from build123d import *
from OCP.BRepFilletAPI import BRepFilletAPI_MakeChamfer

# Parameters (mm, degrees)
SKETCH1_W                = 50
SKETCH1_H                = 21
BOSS_EXTRUDE1_DEPTH      = 2
SKETCH2_W                = 50
SKETCH2_H                = 42
SKETCH2_R                = 2
SKETCH2_R_2              = 12.5
BOSS_EXTRUDE2_DEPTH      = 4
BOSS_EXTRUDE3_START      = -50
BOSS_EXTRUDE3_DEPTH      = 50
CUT_EXTRUDE1_START       = -17
SKETCH4_W                = 46
SKETCH4_H                = 40
CUT_EXTRUDE1_DEPTH       = 17
BOSS_EXTRUDE4_DEPTH      = 8
BOSS_EXTRUDE4_DEPTH_BACK = 8
SKETCH6_R                = 12.5
CUT_EXTRUDE2_DEPTH       = 68.475921631
CHAMFER1_SIZE            = 1
CHAMFER1_SIZE2           = 1.795054936
CHAMFER2_SIZE            = 2


with BuildPart() as part:
    # Sketch1 → Boss-Extrude1 (new body)
    with BuildSketch(Plane(origin=(0, 0, 0), x_dir=(1, 0, 0), z_dir=(0, 1, 0))):
        with Locations((25, 10.5)):
            Rectangle(SKETCH1_W, SKETCH1_H)
        with BuildLine():
            Line((7.25, 11), (7.25, 10))
            ThreePointArc((7.25, 10), (5, 7.75), (2.75, 10))
            Line((2.75, 10), (2.75, 11))
            ThreePointArc((2.75, 11), (5, 13.25), (7.25, 11))
        make_face(mode=Mode.SUBTRACT)
        with BuildLine():
            Line((42.75, 11), (42.75, 10))
            ThreePointArc((42.75, 10), (45, 7.75), (47.25, 10))
            Line((47.25, 10), (47.25, 11))
            ThreePointArc((47.25, 11), (45, 13.25), (42.75, 11))
        make_face(mode=Mode.SUBTRACT)
        with BuildLine():
            Line((27.25, 16), (27.25, 15))
            ThreePointArc((27.25, 15), (25, 12.75), (22.75, 15))
            Line((22.75, 15), (22.75, 16))
            ThreePointArc((22.75, 16), (25, 18.25), (27.25, 16))
        make_face(mode=Mode.SUBTRACT)
    extrude(amount=BOSS_EXTRUDE1_DEPTH)

    # Sketch2 → Boss-Extrude2 (add)
    with BuildSketch(Plane.XY):
        with Locations((25, 21)):
            Rectangle(SKETCH2_W, SKETCH2_H)
        with Locations((9.5, 36.5)):
            Circle(SKETCH2_R, mode=Mode.SUBTRACT)
        with Locations((9.5, 5.5)):
            Circle(SKETCH2_R, mode=Mode.SUBTRACT)
        with Locations((40.5, 5.5)):
            Circle(SKETCH2_R, mode=Mode.SUBTRACT)
        with Locations((40.5, 36.5)):
            Circle(SKETCH2_R, mode=Mode.SUBTRACT)
        with Locations((25, 21)):
            Circle(SKETCH2_R_2, mode=Mode.SUBTRACT)
    extrude(amount=-BOSS_EXTRUDE2_DEPTH)

    # Sketch3 → Boss-Extrude3 (add)
    with BuildSketch(Plane(origin=(50, 0, 0), x_dir=(0, 0, -1), z_dir=(1, 0, 0)).offset(BOSS_EXTRUDE3_START)):
        with BuildLine():
            Line((21, 2), (4, 42))
            Line((4, 42), (4, 2))
            Line((4, 2), (6.5, 2))
            Line((6.5, 2), (6.5, 4))
            ThreePointArc((6.5, 4), (6.939339828, 5.060660172), (8, 5.5))
            Line((8, 5.5), (13, 5.5))
            ThreePointArc((13, 5.5), (14.060660172, 5.060660172), (14.5, 4))
            Line((14.5, 4), (14.5, 2))
            Line((14.5, 2), (21, 2))
        make_face()
    extrude(amount=BOSS_EXTRUDE3_DEPTH)

    # Sketch4 → Cut-Extrude1 (cut)
    with BuildSketch(Plane(origin=(0, 0, -21), x_dir=(-1, 0, 0), z_dir=(0, 0, -1)).offset(CUT_EXTRUDE1_START)):
        with Locations((-25, 22)):
            Rectangle(SKETCH4_W, SKETCH4_H)
    extrude(amount=CUT_EXTRUDE1_DEPTH, mode=Mode.SUBTRACT)

    # Sketch5 → Boss-Extrude4 (add, two sides: drawn at the far end of the back side and taken through both)
    with BuildSketch(Plane.ZY.offset(-25).offset(-BOSS_EXTRUDE4_DEPTH_BACK)):
        Polygon((-4, 2), (-8, 2), (-4, 12), align=None)
    extrude(amount=BOSS_EXTRUDE4_DEPTH + BOSS_EXTRUDE4_DEPTH_BACK)

    # Sketch6 → Cut-Extrude2 (cut, through all)
    with BuildSketch(Plane.XY.offset(-4)):
        with Locations((25, 21)):
            Circle(SKETCH6_R)
    extrude(amount=-CUT_EXTRUDE2_DEPTH, mode=Mode.SUBTRACT)

    # Chamfer1: one chamfer whose edges measure the first distance from different faces: ONE call of the kernel's chamfer builder (chamfer() names one face for all edges)
    chamfer1_edges_1 = [part.edges().sort_by_distance(p)[0] for p in [
        (2, 2, -17.75),
        (48, 2, -17.75),
        (48, 2, -5.25),
        (40.5, 2, -4),
        (2, 2, -5.25),
        (9.5, 2, -4),
        (33, 2, -6),
        (17, 2, -6),
    ]]
    chamfer1_edges_2 = [part.edges().sort_by_distance(p)[0] for p in [
        (25, 2, -8),
    ]]
    chamfer1_side_2 = [part.faces().sort_by_distance(p)[0] for p in [
        (1, 2, -13.971890163),
    ]]
    chamfer1 = BRepFilletAPI_MakeChamfer(part.part.solid().wrapped)
    for e in chamfer1_edges_1:
        chamfer1.Add(CHAMFER1_SIZE, e.wrapped)
    for e in chamfer1_edges_2:
        chamfer1.Add(CHAMFER1_SIZE, CHAMFER1_SIZE2, e.wrapped, chamfer1_side_2[0].wrapped)  # the first distance lies on this face
    add(Compound.cast(chamfer1.Shape()), mode=Mode.REPLACE)

    # Chamfer2
    chamfer2_edges = [part.edges().sort_by_distance(p)[0] for p in [
        (48, 22.5, -4),
        (2, 22.5, -4),
    ]]
    chamfer(chamfer2_edges, length=CHAMFER2_SIZE - 0.0001)  # a hair under: the kernel refuses the full size


solid = part.part
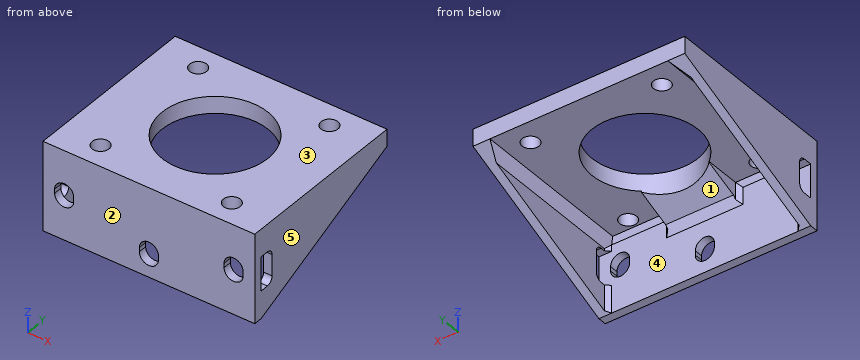
Input: part model. Units: mm. Frame: model coordinates. Face numbers are marked on the shaded views. A direction names the side the tool comes from. Give positions to 0.01 mm unless a question says otherwise; leave off trailing zeros. Order: outer loops, then holes, each group sorted by start corner. A loop starts at its lowest first (then second) coordinate and runs counter-clockwise, first axis right, second up. Notation, with made-up numbers: M 13.25,8 L 62.25,8 A12 cw 62.25,19 Z; hole C 66,4.5 d1. An arc over 180 degrees is marked long. Answer as a JSON object with one key per item and string values.
1. Pull-direction query (X, two-part tool) for the marked faces 3, 4 and 5; classes: +X half, -X half, draft (parallel to the pull), parting line (faces both ways), or undercut.
Result sheet:
{"face 3": "draft", "face 4": "undercut", "face 5": "+X half"}
2. Cut plane A-A, the plane x = 5. Output: boundary loops of the cut face in (y, z), and give its area (4 significant figures).
Result sheet:
{"outline": "M 0,-21 L 2,-21 L 2,-13.25 L 0,-13.25 Z; M 0,-7.75 L 2,-7.75 L 2,-5 L 3,-4 L 42,-4 L 42,0 L 0,0 Z", "area": "191.5 mm²"}
3. Cut plane C-C, the plane y = 36.5. Output: boundary loops of the cut face in (x, z), and give its area (3 significant figures).
Result sheet:
{"outline": "M 0,-6.34 L 2,-6.34 L 2,-6 L 4,-4 L 7.5,-4 L 7.5,0 L 0,0 Z; M 11.5,-4 L 38.5,-4 L 38.5,0 L 11.5,0 Z; M 42.5,-4 L 46,-4 L 48,-6 L 48,-6.34 L 50,-6.34 L 50,0 L 42.5,0 Z", "area": "181 mm²"}
4. Reachability of the marked faces 1 and 2 from +Z, -Z, +X, -X, +Y, -Y: full face, straight path, thin tool, end or side. Return the list, or none.
Result sheet:
{"face 1": "-Z, +Y", "face 2": "+Z, -Z, +X, -X, -Y"}
5. First-contact query: P1, Ø10, axis at x = 8, z = -17, coming from the -Y side; P2, Ø5, axis at x = 33.5, z = -12.5, coming from the +Y side. Flat tips, straight axial feed; report the tip coordinate or a pass-through.
Result sheet:
{"P1": "y = 0", "P2": "y = 2"}
6. Ray query, line 1 (Y direction, x = 9.5, z = -2.55); line 2 (X direction, y = 7, z = -13.75); line 3 (Z direction, x = 3, y = 37). Return the intervals inside material, ascending. Write a range as [from, to].
Result sheet:
{"line 1": "[0, 3.5], [7.5, 34.5], [38.5, 42]", "line 2": "[0, 2], [48, 50]", "line 3": "[-5, 0]"}
7. Cut plane D-D, the plane z = -2.5. Output: boundary loops of the cut face in (x, y), and give its area (3 significant figures).
Result sheet:
{"outline": "M 0,0 L 50,0 L 50,42 L 0,42 Z; hole C 9.5,5.5 d4; hole C 9.5,36.5 d4; hole C 25,21 d25; hole C 40.5,5.5 d4; hole C 40.5,36.5 d4", "area": "1,560 mm²"}
8. Cut plane B-B, the plane x = 25. Output: boundary loops of the cut face in (y, z), and give its area (3 significant figures).
Result sheet:
{"outline": "M 0,-21 L 2,-21 L 2,-18.25 L 0,-18.25 Z; M 0,-12.75 L 2,-12.75 L 2,-9 L 3.67,-7.33 L 8.5,-5.4 L 8.5,0 L 0,0 Z; M 33.5,-4 L 42,-4 L 42,0 L 33.5,0 Z", "area": "109 mm²"}
